Work out the finished part from the listing and answer in its coordinate system (mm). Coordinates: 2 decimals unless noted, no trailing zeros. Order: outer loops, then holes, each group sorted by start corner. A loop starts at its lowest first (then second) coordinate and runs counter-clockwise, first axis right, second up. Notation, with made-up numbers: (-18, 15) -> (0, 15) arc R18 ccw to (0, 44) -> close; hole circle Ø4 at (78.25, 29.5). An arc over 180 degrees is marked (long way). Write item = value, one per line. Start each with the question number.
Q1. Straight lines are drawn through the part: L1, parallel to Y at x = 35, z = 3.5; L2, parallel to X at y = -15.5, z = 0.3; L3, parallel to X at y = -17.5, z = 0.9. For each, find the intervals that lie inside material, in ascending order. Write a range as from..to.
Q2. The part is cut by section B-B, the plane y = 0. Determine the outline of the cut face in (x, z), plus the area to 3 significant figures.
Q3. The part is cut by section D-D, the plane y = 20.5. Determine the outline of the cut face in (x, z).
Q4. The part is cut by section C-C, the plane z = 2.7. Determine the outline of the cut face in (x, y).
Q5. The part is cut by section A-A, the plane x = -35. Determine the outline of the cut face in (y, z).
Q6. A flat-ended cylindrical pin translates along its axis: pin 1 (2.5 mm diameter, centred on x = 35, y = 0, fed in from -Z). Find the tip coordinate at first contact, or state that the pin passes through.
```python
from build123d import *

# Parameters (mm, degrees)
SKETCH1_W           = 140
SKETCH1_H           = 50
SKETCH1_R           = 1.5
SKETCH1_W_2         = 5
SKETCH1_H_2         = 5
BOSS_EXTRUDE1_DEPTH = 5
FILLET1_R           = 10


with BuildPart() as part:
    # Sketch1 → Boss-Extrude1 (new body)
    with BuildSketch(Plane.XY):
        Rectangle(SKETCH1_W, SKETCH1_H)
        with Locations((35, 0)):
            Circle(SKETCH1_R, mode=Mode.SUBTRACT)
        with Locations((-35, 0)):
            Circle(SKETCH1_R, mode=Mode.SUBTRACT)
        with Locations((27.5, 0)):
            Rectangle(SKETCH1_W_2, SKETCH1_H_2, mode=Mode.SUBTRACT)
        with Locations((42.5, 0)):
            Rectangle(SKETCH1_W_2, SKETCH1_H_2, mode=Mode.SUBTRACT)
        with Locations((-42.5, 0)):
            Rectangle(SKETCH1_W_2, SKETCH1_H_2, mode=Mode.SUBTRACT)
        with Locations((-27.5, 0)):
            Rectangle(SKETCH1_W_2, SKETCH1_H_2, mode=Mode.SUBTRACT)
    extrude(amount=BOSS_EXTRUDE1_DEPTH)

    # Fillet1
    fillet1_edges = [part.edges().sort_by_distance(p)[0] for p in [
        (70, -25, 2.5),
        (-70, -25, 2.5),
        (-70, 25, 2.5),
        (70, 25, 2.5),
    ]]
    fillet(fillet1_edges, radius=FILLET1_R)


solid = part.part
```
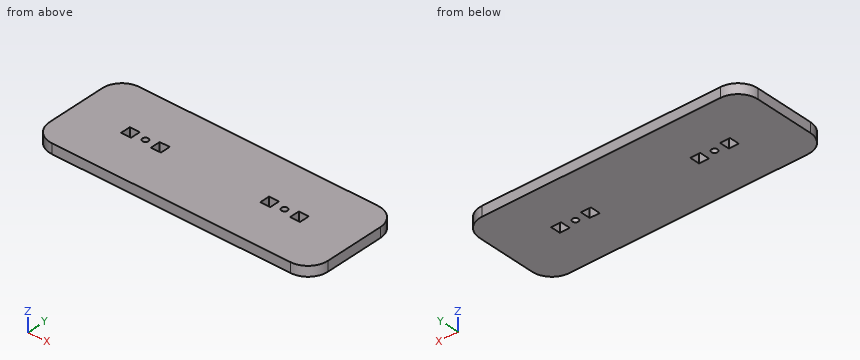
Model answer:
q1.L1 = -25..-1.5, 1.5..25
q1.L2 = -69.99..69.99
q1.L3 = -69.68..69.68
q2.outline = (-70, 0) -> (-45, 0) -> (-45, 5) -> (-70, 5) -> close; (-40, 0) -> (-36.5, 0) -> (-36.5, 5) -> (-40, 5) -> close; (-33.5, 0) -> (-30, 0) -> (-30, 5) -> (-33.5, 5) -> close; (-25, 0) -> (25, 0) -> (25, 5) -> (-25, 5) -> close; (30, 0) -> (33.5, 0) -> (33.5, 5) -> (30, 5) -> close; (36.5, 0) -> (40, 0) -> (40, 5) -> (36.5, 5) -> close; (45, 0) -> (70, 0) -> (70, 5) -> (45, 5) -> close
q2.area = 570 mm2
q3.outline = (-68.35, 0) -> (68.35, 0) -> (68.35, 5) -> (-68.35, 5) -> close
q4.outline = (-70, -15) arc R10 ccw to (-60, -25) -> (60, -25) arc R10 ccw to (70, -15) -> (70, 15) arc R10 ccw to (60, 25) -> (-60, 25) arc R10 ccw to (-70, 15) -> close; hole (-45, -2.5) -> (-40, -2.5) -> (-40, 2.5) -> (-45, 2.5) -> close; hole circle Ø3 at (-35, 0); hole (-30, -2.5) -> (-25, -2.5) -> (-25, 2.5) -> (-30, 2.5) -> close; hole (25, -2.5) -> (30, -2.5) -> (30, 2.5) -> (25, 2.5) -> close; hole circle Ø3 at (35, 0); hole (40, -2.5) -> (45, -2.5) -> (45, 2.5) -> (40, 2.5) -> close
q5.outline = (-25, 0) -> (-1.5, 0) -> (-1.5, 5) -> (-25, 5) -> close; (1.5, 0) -> (25, 0) -> (25, 5) -> (1.5, 5) -> close
q6.pin_1 = through
